from build123d import *

# Parameters (mm, degrees)
SKETCH_W     = 85.4
SKETCH_H     = 123.9
SKETCH_R     = 1.5
PAD_DEPTH    = 2.8
SKETCH001_W  = 2.8
SKETCH001_H  = 25
PAD001_DEPTH = 2.8


with BuildPart() as part:
    # Sketch → Pad (new body)
    with BuildSketch(Plane.XY):
        with Locations((22.7, 49.55)):
            Rectangle(SKETCH_W, SKETCH_H)
        with Locations((8.9, -4)):
            Circle(SKETCH_R, mode=Mode.SUBTRACT)
        with Locations((30.4, -4)):
            Circle(SKETCH_R, mode=Mode.SUBTRACT)
        with Locations((8.9, 102.5)):
            Circle(SKETCH_R, mode=Mode.SUBTRACT)
        with Locations((30.4, 102.5)):
            Circle(SKETCH_R, mode=Mode.SUBTRACT)
        with BuildLine():
            Line((4, 91.5), (45.4, 91.5))
            ThreePointArc((49.4, 87.5), (48.228427, 90.328427), (45.4, 91.5))
            Line((49.4, 87.5), (49.4, 77.5))
            ThreePointArc((47.4, 75.5), (48.814214, 76.085786), (49.4, 77.5))
            Line((47.4, 75.5), (46.3, 75.5))
            ThreePointArc((46.3, 75.5), (44.885786, 74.914214), (44.3, 73.5))
            Line((44.3, 66.3), (44.3, 73.5))
            ThreePointArc((42.3, 64.3), (43.714214, 64.885786), (44.3, 66.3))
            Line((42.1, 64.3), (42.3, 64.3))
            ThreePointArc((42.1, 64.3), (40.685786, 63.714214), (40.1, 62.3))
            Line((40.1, 24.8), (40.1, 62.3))
            ThreePointArc((40.1, 24.8), (41.271573, 21.971573), (44.1, 20.8))
            Line((45.4, 20.8), (44.1, 20.8))
            ThreePointArc((49.4, 16.8), (48.228427, 19.628427), (45.4, 20.8))
            Line((49.4, 16.8), (49.4, 4))
            ThreePointArc((45.4, 0), (48.228427, 1.171573), (49.4, 4))
            Line((45.4, 0), (4, 0))
            ThreePointArc((0, 4), (1.171573, 1.171573), (4, 0))
            Line((0, 4), (0, 87.5))
            ThreePointArc((4, 91.5), (1.171573, 90.328427), (0, 87.5))
        make_face(mode=Mode.SUBTRACT)
    extrude(amount=PAD_DEPTH)

    # Sketch001 → Pad001 (join)
    with BuildSketch(Plane.XY):
        with Locations((14.4, 12.5)):
            Rectangle(SKETCH001_W, SKETCH001_H)
    extrude(amount=PAD001_DEPTH)


solid = part.part
Geometry: final body of the model. Coordinates: model frame, mm. A direction names the side the tool comes from. Round coordinates to 2 decimals unless told otherwise and drop trailing zeros. Loops run counter-clockwise (first coordinate to the right, second up) from the corner with the lowest first, then second, coordinate; pieces in that order, holes last.
Q1. Section A-A on y = 36. Return loops of the section in (x, z).
Q2. Section B-B on x = 8.9. Return loops of the section in (y, z).
Q3. Pin query (flat end, axial travel): P1, Ø12, axis at x = 17.5, y = 23, coming from the -Z side. Return the tip coordinate at first contact, or that it passes through.
Q4. Access query for faces 1 (the cylindrical face through (1.203, 90.359, 1.38)), 2 (the flat face through (65.4, 49, 1)). Directions: +Z, -Z, +X, -X, +Y, -Y. A direction counts if a zero-diameter tool reaches every point of the face in a straight line with its end or side. Return the directions, or none.
Q5. Section D-D on x = 26. Return loops of the section in (y, z), plus the area to 3 significant figures.
Q6. Section C-C on z = 2.2. State how many separate pieces and enclosed holes the cut face has, plus the area to 3 significant figures.
Q7. Material intervals for L1, parallel to Y at x = 30.4, z = 1.65; L2, parallel to X at y = 102.5, z = 1; L3, parallel to X at y = 48.5, z = 0.8, sorted ascending.
Q8. Pull-direction query (Y, two-part tool) for faces 3 (the flat face through (22, 111.5, 1)), 4 (the flat face through (15.8, 12, 1)), 5 (the flat face through (41, 50, 2.8)); classes: released by +Y, released by -Y, zero draft, split by the parting line, or undercut.
Evaluation:
1. outline: (-20, 0) - (0, 0) - (0, 2.8) - (-20, 2.8) - close; (40.1, 0) - (65.4, 0) - (65.4, 2.8) - (40.1, 2.8) - close
2. outline: (-12.4, 0) - (-5.5, 0) - (-5.5, 2.8) - (-12.4, 2.8) - close; (-2.5, 0) - (0, 0) - (0, 2.8) - (-2.5, 2.8) - close; (91.5, 0) - (101, 0) - (101, 2.8) - (91.5, 2.8) - close; (104, 0) - (111.5, 0) - (111.5, 2.8) - (104, 2.8) - close
3. P1: stops at z = 0
4. face 1: +Z, -Z
4. face 2: +Z, -Z, +X, +Y, -Y
5. outline: (-12.4, 0) - (0, 0) - (0, 2.8) - (-12.4, 2.8) - close; (91.5, 0) - (111.5, 0) - (111.5, 2.8) - (91.5, 2.8) - close
5. area: 90.7 mm2
6. separate pieces: 1
6. enclosed holes: 5
6. area: 6,580 mm2
7. L1: y = -12.4 to -5.5, -2.5 to 0, 91.5 to 101, 104 to 111.5
7. L2: x = -20 to 7.4, 10.4 to 28.9, 31.9 to 65.4
7. L3: x = -20 to 0, 40.1 to 65.4
8. face 3: released by +Y
8. face 4: undercut
8. face 5: zero draft
